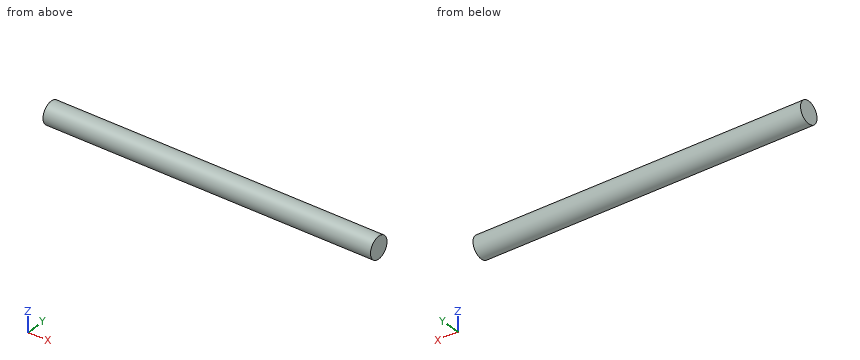
from build123d import *

# Parameters (mm, degrees)
F0_R     = 2.442894711
F1_DEPTH = 58.42
F3_R     = 2.54
F4_DEPTH = 76.2


with BuildPart() as f1:
    # F0 (on Front) → F1 (new body)
    with BuildSketch(Plane.XZ):
        Circle(F0_R)
    extrude(amount=F1_DEPTH)


with BuildPart() as f4:
    # F3 (on Right) → F4 (new body)
    with BuildSketch(Plane.YZ):
        Circle(F3_R)
    extrude(amount=F4_DEPTH)


solid = f4.part
For this review, take the finished solid that the model builds, in its own axes (mm). Give positions to 0.01 mm unless a question says otherwise; leave off trailing zeros. Loops run counter-clockwise (first coordinate to the right, second up) from the corner with the lowest first, then second, coordinate; pieces in that order, holes last. Notation, with made-up numbers: M 12.25,-3.5 L 41.25,-3.5 A20 ccw 41.25,7.5 Z; hole C 43,47.25 d5. An arc over 180 degrees is marked long. Answer as a JSON object with one key per item and string values. Group by question number.
Q1. Add section A-A on x = 26.5. Give the boundary of the cut face in (y, z).
Q2. Add section B-B on y = 0.75. Give the boundary of the cut face in (x, z), and give its area (3 significant figures).
Q3. Add section C-C on z = -0.65. Give the boundary of the cut face in (x, y).
Q4. Insertion check: P1, Ø1, axis at x = 34, z = 1, coming from the +Y side. The pin has a flat end and moves straight along its axis. Give the tip position at first contact, or say it passes through.
Q5. For probe 1 along Z at (x, y) = (62, -0.2); probe 2 along Z at (x, y) = (31, -0.75), list the stretches that pass through material, from the lowest coordinate up. Write a range as [from, to].
Checked values:
{
 "1": {"outline": "C 0,0 d5.08"},
 "2": {"outline": "M 0,-2.43 L 76.2,-2.43 L 76.2,2.43 L 0,2.43 Z", "area": "370 mm²"},
 "3": {"outline": "M 0,-2.46 L 76.2,-2.46 L 76.2,2.46 L 0,2.46 Z"},
 "4": {"P1": "y = 2.49"},
 "5": {"probe 1": "[-2.53, 2.53]", "probe 2": "[-2.43, 2.43]"}
}
